from build123d import *

# Parameters (mm, degrees)
F0_R     = 11
F1_DEPTH = 12.5
F2_SIZE  = 12
F3_R     = 10
F4_SIZE  = 12


# Not quite as in the source:
# - a feature names something its author has since deleted; it is built from what else it names


with BuildPart() as f1:
    # F0 (on Right) → F1 (new body, symmetric)
    with BuildSketch(Plane.YZ):
        with BuildLine():
            Line((-108.2477509669, 143.9956215311), (-146.1053743867, -65.5600531085))
            Line((-146.1053743867, -65.5600531085), (0, -65.5600531085))
            Line((0, -65.5600531085), (146.1053743867, -65.5600531085))
            Line((146.1053743867, -65.5600531085), (108.2477509669, 143.9956215311))
            ThreePointArc((108.2477509669, 143.9956215311), (0, 234.4399468915), (-108.2477509669, 143.9956215311))
        make_face()
        with BuildLine():
            Line((-85.1559906377, -42.7505690663), (-69.6519457463, 43.0699419263))
            ThreePointArc((-69.6519457463, 43.0699419263), (0, 17.3303242879), (69.6519457463, 43.0699419263))
            Line((69.6519457463, 43.0699419263), (85.1559906377, -42.7505690663))
            Line((85.1559906377, -42.7505690663), (0, -42.7505690663))
            Line((0, -42.7505690663), (-85.1559906377, -42.7505690663))
        make_face(mode=Mode.SUBTRACT)
        with BuildLine():
            ThreePointArc((56.1396103068, 74.707219693), (0, 49.4399468915), (-56.1396103068, 74.707219693))
            Line((-56.1396103068, 74.707219693), (-15, 98.459184778))
            ThreePointArc((-15, 98.459184778), (0, 94.4399468915), (15, 98.459184778))
            Line((15, 98.459184778), (56.1396103068, 74.707219693))
        make_face(mode=Mode.SUBTRACT)
        with BuildLine():
            Line((-15, 197.924639175), (-15, 150.420709005))
            ThreePointArc((-15, 150.420709005), (-25.9807621135, 139.4399468915), (-30, 124.4399468915))
            Line((-30, 124.4399468915), (-71.1396103068, 100.6879818065))
            ThreePointArc((-71.1396103068, 100.6879818065), (-64.9519052838, 161.9399468915), (-15, 197.924639175))
        make_face(mode=Mode.SUBTRACT)
        with Locations((0, 124.4399468915)):
            Circle(F0_R, mode=Mode.SUBTRACT)
        with BuildLine():
            Line((15, 150.420709005), (15, 197.924639175))
            ThreePointArc((15, 197.924639175), (64.9519052838, 161.9399468915), (71.1396103068, 100.6879818065))
            Line((71.1396103068, 100.6879818065), (30, 124.4399468915))
            ThreePointArc((30, 124.4399468915), (25.9807621135, 139.4399468915), (15, 150.420709005))
        make_face(mode=Mode.SUBTRACT)
    extrude(amount=F1_DEPTH, both=True)

    # F2
    f2_edges = [f1.edges().sort_by_distance(p)[0] for p in [
        (12.5, 0, 234.439947),
    ]]
    chamfer(f2_edges, length=F2_SIZE)

    # F3
    f3_edges = [f1.edges().sort_by_distance(p)[0] for p in [
        (0, -69.651946, 43.069942),
        (0, 69.651946, 43.069942),
        (0, -85.155991, -42.750569),
        (0, 85.155991, -42.750569),
        (0, -15, 197.924639),
        (0, 15, 197.924639),
        (0, -71.13961, 100.687982),
        (0, -56.13961, 74.70722),
        (0, 56.13961, 74.70722),
        (0, 71.13961, 100.687982),
    ]]
    fillet(f3_edges, radius=F3_R)

    # F4
    f4_edges = [f1.edges().sort_by_distance(p)[0] for p in [
        (12.5, 0, 17.330324),
        (12.5, -64.951905, 161.939947),
        (12.5, 64.951905, 161.939947),
        (12.5, 0, 49.439947),
        (12.5, -25.980762, 139.439947),
        (12.5, 0, 94.439947),
        (12.5, 25.980762, 139.439947),
    ]]
    chamfer(f4_edges, length=F4_SIZE)


solid = f1.part
Input: part model. Units: mm. Frame: model coordinates. A direction names the side the tool comes from. Give positions to 0.01 mm unless a question says otherwise; leave off trailing zeros. Order: outer loops, then holes, each group sorted by start corner. A loop starts at its lowest first (then second) coordinate and runs counter-clockwise, first axis right, second up. Notation, with made-up numbers: (64, 54.5) - (116, 54.5) arc R32 ccw to (116, 91.5) - close; hole circle Ø4 at (23.5, 85.5). An arc over 180 degrees is marked (long way). Answer as a JSON object with one key per item and string values. Group by question number.
Q1. First-contact query: pin 1 Ø2 at (x, z) = (2, 85) entering from -Y; pin 2 Ø1.5 at (y, z) = (83, 134.5) entering from +X; pin 3 Ø1.5 at (x, z) = (8.5, 42) entering from -Y. Flat tips, straight axial feed; report the tip coordinate or a pass-through.
Q2. Cut plane B-B, the plane y = -113. Output: boundary loops of the cut face in (x, z).
Q3. Cut plane A-A, the plane x = -3.25. Count the separate pieces of the cut face and the enclosed holes in it, then the cut area to 3 significant figures.
Q4. Cut plane C-C, the plane y = 112. Output: boundary loops of the cut face in (x, z), then the cut area to 3 significant figures.
Q5. Mould query, pull axis Y, two halves, no side actions, for faces 4 (the face through (-5.91, -25.87, 139.63)), 5 (the face through (-5.91, 2.14, 234.42)), 6 (the face through (-6.09, 80.78, -39.26)), 7 (the face through (6.584, -120.924, 39.603)). Classes: pulls with the +Y half, pulls with the -Y half, needs draft (parallel to the pull), parting line crosses it, or undercut.
Q6. Set-up query: faces 1 (the face through (-5.909, -126.912, 40.685)), 2 (the face through (-5.909, -66.808, 34.606)), 3 (the face through (7.92, 19.69, 135.49)). Return all of +Z, -Z, +X, -X, +Y, -Y with unobstructed straight access to the full face (end or side cutting, diameter ignored); none if empty.
Q7. Line query: probe 1 along Z at (x, y) = (-4, 0); probe 2 along Z at (x, y) = (-10.5, 62); probe 3 along Y at (x, z) = (6.75, 187.5). Output: solid intervals per line, ascending.
Results:
{
 "1": {"pin 1": "y = -118.41", "pin 2": "x = 9.86", "pin 3": "y = -119.32"},
 "2": {"outline": "(-12.5, -65.56) - (12.5, -65.56) - (12.5, 50.19) - (0.5, 117.69) - (-12.5, 117.69) - close"},
 "3": {"separate pieces": "1", "enclosed holes": "5", "area": "46,500 mm^2"},
 "4": {"outline": "(-12.5, -65.56) - (12.5, -65.56) - (12.5, 55.73) - (0.5, 123.23) - (-12.5, 123.23) - close", "area": "4,310 mm^2"},
 "5": {"face 4": "undercut", "face 5": "parting line crosses it", "face 6": "undercut", "face 7": "pulls with the -Y half"},
 "6": {"face 1": "+Z, +X, -X, -Y", "face 2": "+X, -X", "face 3": "+X"},
 "7": {"probe 1": "-65.56 to -42.75, 17.33 to 49.44, 94.44 to 113.44, 135.44 to 234.44", "probe 2": "-65.56 to -42.75, 35.48 to 106.4, 166.64 to 215.3", "probe 3": "-82.39 to -51.23, -9.04 to 9.04, 51.23 to 82.39"}
}
